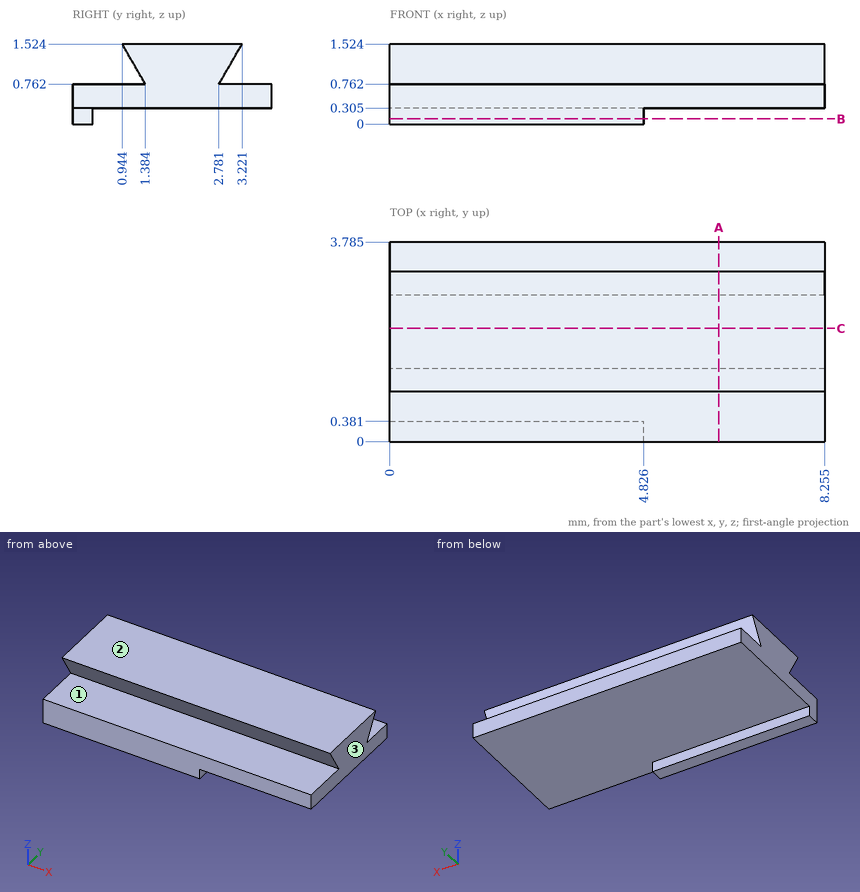
Could you check a few things on this drawing? It's one solid part, dimensions in mm from its lowest x, y, z. Coordinates: 2 decimals unless noted, no trailing zeros. Order: outer loops, then holes, each group sorted by start corner. A loop starts at its lowest first (then second) coordinate and runs counter-clockwise, first axis right, second up. Notation, with made-up numbers: M 43.5,64 L 55.5,64 A27 ccw 55.5,89 Z; hole C 27,-6 d5. An arc over 180 degrees is marked long. Use a Markdown table: item, result. Add a question column.
Q1. If I drill on L1, parallel to Z at x = 5, y = 2.2 (1 decimal); L2, parallel to Y at x = 2.25, z = 0.2; L3, parallel to Z at x = 0.5, y = 0.2, over which ranges is the centre line in solid material (lowest first)?
Q2. I want a section at B-B on z = 0.1. List the corners of the cut face in (x, y) for me.
Q3. I'm going to push a flat-ended pin straight in: pin 1 (1.1 mm diameter, centred on x = 5, y = 2, fed in from -Z) (1 decimal). Where does the tip first touch, or does it pass through?
Q4. I want a section at A-A on x = 6.25. List the corners of the cut face in (y, z) for me (1 decimal).
Q5. I want a section at C-C on y = 2.15. List the corners of the cut face in (x, z) for me (1 decimal).
Q6. We'd pull the mould along Z, two halves only. Please class the marked faces 1, 2 and 3: pulls with the +Z half, pulls with the -Z half, needs draft (parallel to the pull), parting line crosses it, or undercut.
Checked values:
| question | item | result |
|---|---|---|
| 1 | L1 | 0.3 to 1.5 |
| 1 | L2 | 0 to 0.38 |
| 1 | L3 | 0 to 0.76 |
| 2 | outline | M 0,0 L 4.83,0 L 4.83,0.38 L 0,0.38 Z |
| 3 | pin 1 | z = 0.3 |
| 4 | outline | M 0,0.3 L 3.8,0.3 L 3.8,0.8 L 2.8,0.8 L 3.2,1.5 L 0.9,1.5 L 1.4,0.8 L 0,0.8 Z |
| 5 | outline | M 0,0.3 L 8.3,0.3 L 8.3,1.5 L 0,1.5 Z |
| 6 | face 1 | undercut |
| 6 | face 2 | pulls with the +Z half |
| 6 | face 3 | needs draft |
